Autodesk Inventor part; units mm, degrees
ref_plane "YZ Plane" through (0, 0, 0) normal (1, 0, 0) x (0, 1, 0)
ref_plane "XZ Plane" through (0, 0, 0) normal (0, 1, 0) x (-1, 0, 0)
ref_plane "XY Plane" through (0, 0, 0) normal (0, 0, 1) x (1, 0, 0)
sketch "Sketch1" plane through (0, 0, 0) normal (0, 1, 0) x (-1, 0, 0)
  circle A0 centre (0, 0) radius 1.5
  circle A1 centre (0, 0) radius 4.5
  line L0 (-1.6021, 2.775) -> (1.6021, 2.775)
  line L1 (1.6021, 2.775) -> (3.2043, 0)
  line L2 (3.2043, 0) -> (1.6021, -2.775)
  line L3 (1.6021, -2.775) -> (-1.6021, -2.775)
  line L4 (-1.6021, -2.775) -> (-3.2043, 0)
  line L5 (-3.2043, 0) -> (-1.6021, 2.775)
  line L6 (6.3, 0) -> (-6.3, 0)
  dimension "d0" = 3
  dimension "d1" = 9
  dimension "d2" = 5.55
extrude "Extrusion1" add sketch "Sketch1" along normal blind 3.3 contours L6 A1 L4 L3 L2 | L1 L0 L5 L6 A1
sketch "Sketch2" plane through (0, 3.3, 0) normal (0, 1, 0) x (1, 0, 0)
  line L0 (-1.6021, -2.775) -> (-3.2043, 0)
  line L1 (-3.2043, 0) -> (-1.6021, 2.775)
  line L2 (-1.6021, 2.775) -> (1.6021, 2.775)
  line L3 (1.6021, 2.775) -> (3.2043, 0)
  line L4 (3.2043, 0) -> (1.6021, -2.775)
  line L5 (1.6021, -2.775) -> (-1.6021, -2.775)
  circle A0 centre (0, 0) radius 4.5
  circle A1 centre (0, 0) radius 1.5
  dimension "d5" = 3
extrude "Extrusion2" add sketch "Sketch2" along normal blind 2 contours L0 L1 L2 L3 L4 L5 | A0
sketch "Sketch3" plane through (0, 0, 0) normal (0, -1, 0) x (1, 0, 0)
  point P0 (0, 0)
sketch "Sketch4" plane through (0, 0, 0) normal (0, -1, 0) x (1, 0, 0)
  line L0 (-3.2043, 0) -> (-1.6021, 2.775)
  line L1 (-1.6021, 2.775) -> (1.6021, 2.775)
  line L2 (1.6021, 2.775) -> (3.2043, 0)
  line L3 (3.2043, 0) -> (1.6021, -2.775)
  line L4 (1.6021, -2.775) -> (-1.6021, -2.775)
  line L5 (-1.6021, -2.775) -> (-3.2043, 0)
  circle A0 centre (0, 0) radius 4.5
  line L6 (3.5218, 0) -> (1.7609, 3.05)
  line L7 (1.7609, 3.05) -> (-1.7609, 3.05)
  line L8 (-1.7609, 3.05) -> (-3.5218, 0)
  line L9 (-3.5218, 0) -> (-1.7609, -3.05)
  line L10 (-1.7609, -3.05) -> (1.7609, -3.05)
  line L11 (1.7609, -3.05) -> (3.5218, 0)
  dimension "d8" = 6.1
extrude "Extrusion3" add sketch "Sketch4" along normal blind 4 contours A0
properties part number "30_Adapter_M3_nut"
Work out the finished part from the listing and answer in its coordinate system (mm). A direction names the side the tool comes from. Give positions to 0.01 mm unless a question says otherwise; leave off trailing zeros. Write each loop counter-clockwise with the first axis right and the second up, starting at its lowest first coordinate (ties: lowest second). Pieces come first, ordered by that corner, then holes. Notation, with made-up numbers: (40.25, 43.25) - (94.25, 43.25) arc R13 ccw to (94.25, 62.25) - close; hole circle Ø5 at (-6.75, -1). An arc over 180 degrees is marked (long way). One line per item, written item: value. Start each with the question number.
1. Consider probe 1 along Z at (x, y) = (0, 4.65); probe 2 along Y at (x, z) = (-2.75, 1). Determine where each line is inside the solid, lowest interval first.
2. For a pull along X with two mould halves and no side action, classify faces 3 (the flat face through (-2.629, -1.972, 1.546)), 4 (the flat face through (0, 5.3, 2)), 5 (the flat face through (-2.414, 1.627, -1.368)) as +X half, -X half, draft (parallel to the pull), parting line (faces both ways), or undercut.
3. Given pin 1 (1 mm diameter, centred on x = 3, y = -1, fed in from +Z); pin 2 (4 mm diameter, centred on x = 0.5, z = 0, fed in from -Y); pin 3 (4 mm diameter, centred on x = -3.5, y = 1, fed in from -Z), each flat-ended and moving along its own axis, determine where each tip first touches the part or whether it passes through.
4. For faces 1 (the flat face through (-3.1, -4, 1.1)), 2 (the flat face through (2.39, 1.63, -1.41)), determine the directions among +Z, -Z, +X, -X, +Y, -Y from which every point of the face is accessible in a straight line to the end or side of a thin tool.
5. Find section A-A (y = 1.75). Write down the section's boundary in (x, z) (3 decimals), then the cut area to 3 significant figures.
6. Find section C-C (y = -2.5). Write down the section's boundary in (x, z), then the cut area to 3 significant figures.
Geometry results:
1. probe 1: -4.5 to -1.5, 1.5 to 4.5
1. probe 2: 0 to 5.3
2. face 3: undercut
2. face 4: draft
2. face 5: undercut
3. pin 1: z = 3.74
3. pin 2: y = 3.3
3. pin 3: z = -4.24
4. face 1: +Z, -Z, +X, -X, -Y
4. face 2: -Y
5. outline: circle Ø9 at (0, 0); hole (-3.204, 0) - (-1.602, -2.775) - (1.602, -2.775) - (3.204, 0) - (1.602, 2.775) - (-1.602, 2.775) - close
5. area: 36.9 mm2
6. outline: circle Ø9 at (0, 0); hole (-3.52, 0) - (-1.76, -3.05) - (1.76, -3.05) - (3.52, 0) - (1.76, 3.05) - (-1.76, 3.05) - close
6. area: 31.4 mm2
